Design review of the part shown in the three views and the two pictorial views. Dimensions are in mm from the part's minimum x, y and z. Coordinates: 2 decimals unless noted, no trailing zeros. Write each loop counter-clockwise with the first axis right and the second up, starting at its lowest first coordinate (ties: lowest second). Pieces come first, ordered by that corner, then holes. Notation, with made-up numbers: (1.5, -23.75) - (52.5, -23.75) arc R16 ccw to (52.5, -7.75) - close; hole circle Ø4 at (-30, 61.5). An arc over 180 degrees is marked (long way). Write each question's results on one line, items separated by ' | '.
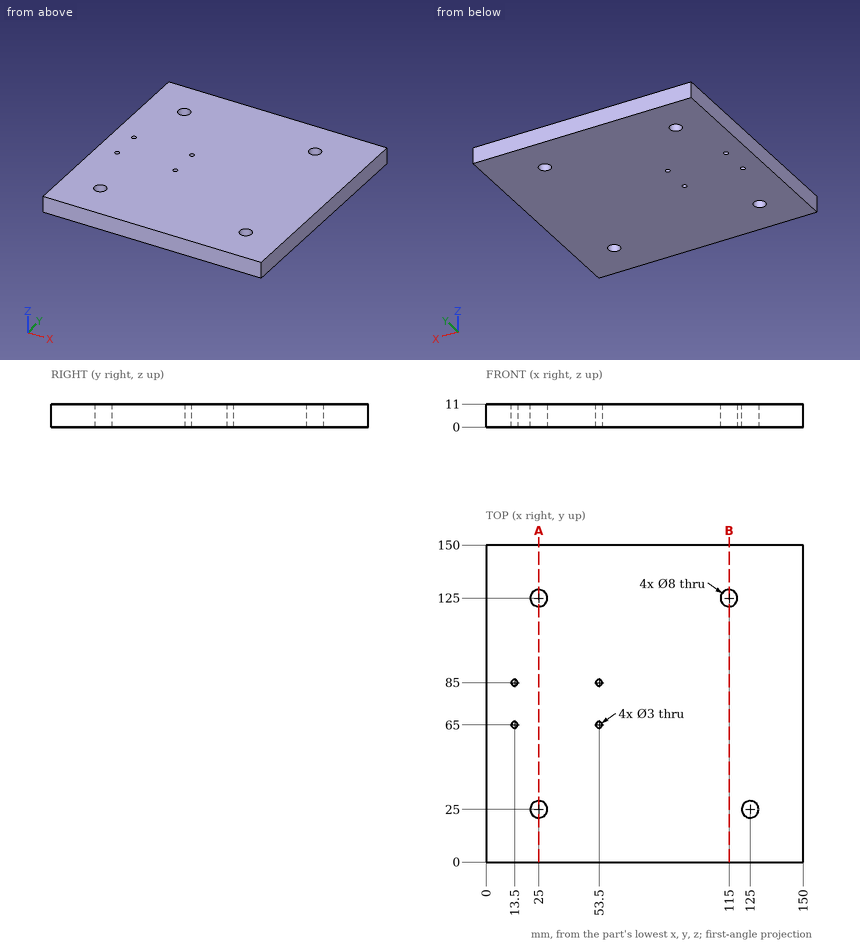
Q1. Take a section at A-A on x = 25. State the section outline as (y, z) points.
Results found:
outline: (0, 0) - (21, 0) - (21, 11) - (0, 11) - close; (29, 0) - (121, 0) - (121, 11) - (29, 11) - close; (129, 0) - (150, 0) - (150, 11) - (129, 11) - close
Q2. For pin 1 (7 mm diameter, centred on x = 25, y = 125, fed in from -Z), flat-tipped, find the tip position at first contact; note if it passes through.
Results found:
pin 1: through
Q3. Take a section at B-B on x = 115. State the section outline as (y, z) points, plus the area to 3 significant figures.
Results found:
outline: (0, 0) - (121, 0) - (121, 11) - (0, 11) - close; (129, 0) - (150, 0) - (150, 11) - (129, 11) - close | area: 1,560 mm2
Q4. Wall thickness on line 1 along X through (y, z) = (65, 3.25); line 2 along Y through (x, z) = (25, 6.25); line 3 along Y through (x, z) = (53.5, 4.75): over which ranges is each line inside the solid? List them lowest first. Write a range as from..to.
Results found:
line 1: 0..12, 15..52, 55..150 | line 2: 0..21, 29..121, 129..150 | line 3: 0..63.5, 66.5..83.5, 86.5..150
